Design review of the part built by this model. Coordinates are the model's own, in mm. Face numbers are marked on the shaded views. A direction names the side the tool comes from. Coordinates: 2 decimals unless noted, no trailing zeros. Loops run counter-clockwise (first coordinate to the right, second up) from the corner with the lowest first, then second, coordinate; pieces in that order, holes last. Notation, with made-up numbers: M 49.25,41 L 106.25,41 A22 cw 106.25,56 Z; hole C 24,-25.5 d10. An arc over 180 degrees is marked long. Put each result on its own line as item: value. Start each with the question number.
(1) Clearance check with flat-ended pins moving along their axes: pin 1 (8 mm diameter, centred on x = 36.5, y = 3.5, fed in from +Z); pin 2 (4 mm diameter, centred on x = 6, y = -39, fed in from +Z); pin 3 (8 mm diameter, centred on x = 12, y = -34.5, fed in from -Z); pin 4 (5 mm diameter, centred on y = 0, z = 0, fed in from +X). State where each tip first meets the part, or that it passes through.
(2) For probe 1 along X at (y, z) = (-9, 42.5); probe 2 along Z at (x, y) = (4, -31); probe 3 along X at (y, z) = (-6, 9), list the stretches that pass through material, from the lowest coordinate up. Write a range as [from, to].
(3) The part is to be moulded in two halves that separate along Y. For the marked faces 3, 4 and 5, say which applies: +Y half, -Y half, draft (parallel to the pull), parting line (faces both ways), or undercut.
(4) For the marked faces 1 and 2, list the 3-axis set-ups (+Z, -Z, +X, -X, +Y, -Y) from which the entire face can be reached by the end or side of a thin tool; tool diameter is ignored.
(5) Take a section at D-D, the plane x = 32.5. Give the boundary of the cut face in (y, z).
(6) Take a section at C-C, the plane x = 21. Give the boundary of the cut face in (y, z), then the cut area to 3 significant figures.
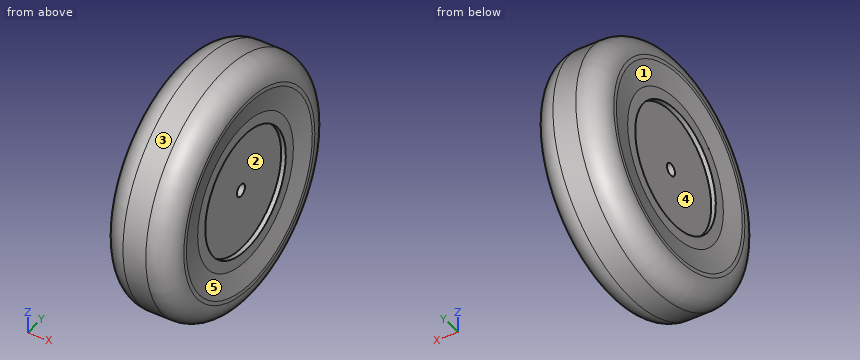
Autodesk Inventor part; units mm, degrees
ref_plane "YZ Plane" through (0, 0, 0) normal (1, 0, 0) x (0, 1, 0)
ref_plane "XZ Plane" through (0, 0, 0) normal (0, 1, 0) x (-1, 0, 0)
ref_plane "XY Plane" through (0, 0, 0) normal (0, 0, 1) x (1, 0, 0)
sketch "Sketch1" plane through (0, 0, 0) normal (1, 0, 0) x (0, 1, 0)
  circle A0 centre (0, 0) radius 80
  dimension "d0" = 160
extrude "Extrusion1" add sketch "Sketch1" along normal blind 45
fillet "Fillet1" radius 15 2 edges at (45, -80, 0) (0, -80, 0)
sketch "Sketch2" plane through (45, 0, 0) normal (1, 0, 0) x (0, 0, -1)
  circle A0 centre (0, 0) radius 47.5
  dimension "d4" = 95
extrude "Extrusion2" cut sketch "Sketch2" against normal blind 2.5
sketch "Sketch3" plane through (0, 0, 0) normal (-1, 0, 0) x (0, 0, 1)
  circle A0 centre (0, 0) radius 47.5
  dimension "d7" = 95
extrude "Extrusion3" cut sketch "Sketch3" against normal blind 2.5
sketch "Sketch4" plane through (42.5, 0, 0) normal (1, 0, 0) x (0, 0, -1)
  circle A0 centre (0, 0) radius 40
  dimension "d10" = 80
extrude "Extrusion4" cut sketch "Sketch4" against normal blind 3
sketch "Sketch5" plane through (2.5, 0, 0) normal (-1, 0, 0) x (0, 0, 1)
  circle A0 centre (0, 0) radius 40
  dimension "d13" = 80
extrude "Extrusion5" cut sketch "Sketch5" against normal blind 3
chamfer "Chamfer1" distance 15 distance2 2.5 1 edges at (0, 0, -47.5) measured on face at (0, 35.0738, -47.3752)
chamfer "Chamfer2" distance 15 distance2 2.5 1 edges at (45, 0, 47.5) measured on face at (45, 35.0738, 47.3752)
sketch "Sketch6" plane through (5.5, 0, 0) normal (-1, 0, 0) x (0, 0, 1)
  circle A0 centre (0, 0) radius 4
  dimension "d22" = 8
extrude "Extrusion6" cut sketch "Sketch6" against normal blind 34000
properties part number "Wheel"
Computed values:
1. pin 1: stops at z = 79.73
1. pin 2: stops at z = 68.29
1. pin 3: stops at z = -73.76
1. pin 4: passes through
2. probe 1: x = [2.5, 42.5]
2. probe 2: z = [-68.51, -25.28], [25.28, 68.51]
2. probe 3: x = [5.5, 39.5]
3. face 3: parting line
3. face 4: undercut
3. face 5: undercut
4. face 1: -X
4. face 2: +X
5. outline: C 0,0 d159.58; hole C 0,0 d8
6. outline: C 0,0 d160; hole C 0,0 d8
6. area: 20,100 mm^2
